```python
from build123d import *

# Parameters (mm, degrees)
SKETCH1_R           = 2.1
BOSS_EXTRUDE1_DEPTH = 65
SKETCH84_W          = 0.3
SKETCH84_H          = 5.4
BOSS_EXTRUDE6_DEPTH = 430
SKETCH85_W          = 26.589814492
SKETCH85_H          = 26.977421118
CUT_EXTRUDE59_DEPTH = 434.070721707
SKETCH86_W          = 10.5
SKETCH86_H          = 16.670499862
CUT_EXTRUDE60_DEPTH = 20
SKETCH88_W          = 63.871976351
SKETCH88_H          = 27.184970046
CUT_EXTRUDE62_DEPTH = 215
BOSS_EXTRUDE7_DEPTH = 195


with BuildPart() as part:
    # Sketch1 → Boss-Extrude1 (new body)
    with BuildSketch(Plane(origin=(0, 0, 0), x_dir=(0, 0, -1), z_dir=(1, 0, 0))):
        with BuildLine():
            Line((-10, 9), (-10, 3))
            Line((-10, 3), (-8, 3))
            Line((-8, 3), (-8, 6))
            Line((-8, 6), (-7.060660172, 6))
            Line((-7.060660172, 6), (-4, 2.939339828))
            Line((-4, 2.939339828), (-4, -2.939339828))
            Line((-4, -2.939339828), (-7.060660172, -6))
            Line((-7.060660172, -6), (-8, -6))
            Line((-8, -6), (-8, -3))
            Line((-8, -3), (-10, -3))
            Line((-10, -3), (-10, -9))
            ThreePointArc((-10, -9), (-9.707106781, -9.707106781), (-9, -10))
            Line((-9, -10), (-3, -10))
            Line((-3, -10), (-3, -8))
            Line((-3, -8), (-6, -8))
            Line((-6, -8), (-6, -7.060660172))
            Line((-6, -7.060660172), (-2.939339828, -4))
            Line((-2.939339828, -4), (2.939339828, -4))
            Line((2.939339828, -4), (6, -7.060660172))
            Line((6, -7.060660172), (6, -8))
            Line((6, -8), (3, -8))
            Line((3, -8), (3, -10))
            Line((3, -10), (9, -10))
            ThreePointArc((9, -10), (9.707106781, -9.707106781), (10, -9))
            Line((10, -9), (10, -3))
            Line((10, -3), (8, -3))
            Line((8, -3), (8, -6))
            Line((8, -6), (7.060660172, -6))
            Line((7.060660172, -6), (4, -2.939339828))
            Line((4, -2.939339828), (4, 2.939339828))
            Line((4, 2.939339828), (7.060660172, 6))
            Line((7.060660172, 6), (8, 6))
            Line((8, 6), (8, 3))
            Line((8, 3), (10, 3))
            Line((10, 3), (10, 9))
            ThreePointArc((10, 9), (9.707106781, 9.707106781), (9, 10))
            Line((9, 10), (3, 10))
            Line((3, 10), (3, 8))
            Line((3, 8), (6, 8))
            Line((6, 8), (6, 7.060660172))
            Line((6, 7.060660172), (2.939339828, 4))
            Line((2.939339828, 4), (-2.939339828, 4))
            Line((-2.939339828, 4), (-6, 7.060660172))
            Line((-6, 7.060660172), (-6, 8))
            Line((-6, 8), (-3, 8))
            Line((-3, 8), (-3, 10))
            Line((-3, 10), (-9, 10))
            ThreePointArc((-9, 10), (-9.707106781, 9.707106781), (-10, 9))
        make_face()
        Circle(SKETCH1_R, mode=Mode.SUBTRACT)
    extrude(amount=BOSS_EXTRUDE1_DEPTH)

    # Sketch85 → Cut-Extrude59 (cut, through all)
    with BuildSketch(Plane(origin=(65, 0, 0), x_dir=(0, 0, -1), z_dir=(1, 0, 0))):
        with Locations((1.176321583, -0.814927094)):
            Rectangle(SKETCH85_W, SKETCH85_H)
    extrude(amount=-CUT_EXTRUDE59_DEPTH, mode=Mode.SUBTRACT)


with BuildPart() as body_2:
    # Sketch84 → Boss-Extrude6 (new body)
    with BuildSketch(Plane(origin=(65, 0, 0), x_dir=(0, 0, -1), z_dir=(1, 0, 0))):
        Polygon((-10, -2.7), (-10, 2.7), (-10.5, 2.7), (-10.5, 5), (-20.5, 5), (-20.5, 0), (-40.5, 0), (-40.5, 5), (-50.5, 5), (-50.5, -5), (-10.5, -5), (-10.5, -2.7), align=None)
        Polygon((-7.18492424, 5.7), (-4.3, 2.81507576), (-4.3, -2.81507576), (-7.18492424, -5.7), (-7.7, -5.7), (-7.7, -2.7), (-9.7, -2.7), (-9.7, 2.7), (-7.7, 2.7), (-7.7, 5.7), align=None)
        with Locations((-9.85, 0)):
            Rectangle(SKETCH84_W, SKETCH84_H)
    extrude(amount=BOSS_EXTRUDE6_DEPTH)

    # Sketch86 → Cut-Extrude60 (cut)
    with BuildSketch(Plane.ZY.offset(-65)):
        with Locations((5.25, -0.117074477)):
            Rectangle(SKETCH86_W, SKETCH86_H)
    extrude(amount=-CUT_EXTRUDE60_DEPTH, mode=Mode.SUBTRACT)

    # Sketch88 → Cut-Extrude62 (cut)
    with BuildSketch(Plane(origin=(495, 0, 0), x_dir=(0, 0, -1), z_dir=(1, 0, 0))):
        with Locations((-29.280082041, 0.441796331)):
            Rectangle(SKETCH88_W, SKETCH88_H)
    extrude(amount=-CUT_EXTRUDE62_DEPTH, mode=Mode.SUBTRACT)

    # Sketch89 → Boss-Extrude7 (add)
    with BuildSketch(Plane(origin=(280, 0, 0), x_dir=(0, 0, -1), z_dir=(1, 0, 0))):
        Polygon((-10.7, 2.9), (-10.7, -2.9), (-7.9, -2.9), (-7.9, -5.9), (-7.102081528, -5.9), (-4.1, -2.897918472), (-4.1, 2.897918472), (-7.102081528, 5.9), (-7.9, 5.9), (-7.9, 2.9), align=None)
        Polygon((-10.5, 2.7), (-10.5, -2.7), (-7.7, -2.7), (-7.7, -5.7), (-7.18492424, -5.7), (-4.3, -2.81507576), (-4.3, 2.81507576), (-7.18492424, 5.7), (-7.7, 5.7), (-7.7, 2.7), align=None, mode=Mode.SUBTRACT)
    extrude(amount=-BOSS_EXTRUDE7_DEPTH)


solid = body_2.part
```
Build history of the part. All positions in model axes, mm. A direction names the side the tool comes from. Give positions to 0.01 mm unless a question says otherwise; leave off trailing zeros. Order: outer loops, then holes, each group sorted by start corner. A loop starts at its lowest first (then second) coordinate and runs counter-clockwise, first axis right, second up. Notation, with made-up numbers: M 61.25,32 L 120.25,32 A27 cw 120.25,49 Z; hole C 20,88.25 d5. An arc over 180 degrees is marked long. Write item = value, one per line. Start each with the question number.
(1) Slice it at C-C on z = 15. Write the cut outline in (x, y).
(2) Slice it at A-A on x = 133. Write the cut outline in (y, z).
(3) Slice it at B-B on z = 32.5. Write the cut outline in (x, y).
(4) Which spindle directions (+Z, -Z, +X, -X, +Y, -Y) get a long thin tool onto all of the face, cutting with end or side? Do faces 4 (the flat face through (171, 3, 20.5)), 5 (the flat face through (85, 0, 7)), 6 (the flat face through (171, 5, 15)). Say none if no direction does.
(5) Probe L1, parallel to Z at x = 166, y = 4; L2, parallel to Z at x = 240, y = 3; L3, parallel to Y at x = 106.5, z = 19. List the from-to ranges inside material, lowest first. Write a range as [from, to].
(6) Pin check, flat tips, straight feed: pin 1 Ø3 at (x, z) = (226, 46.5) entering from +Y; pin 2 Ø2 at (y, z) = (0.5, 36) entering from +X; pin 3 Ø1.5 at (x, z) = (94.5, 25) entering from -Y. Stop position of each tip, or through.
(7) Two-plate mould, pull along Z, no slides. Class faces 1 (the flat face through (65, -1, 31)), 2 (the flat face through (171, 2, 40.5)), 3 (the flat face through (184, 0, 4.1)): released by +Z, released by -Z, zero draft, split by the parting line, or undercut.
Responses:
q1.outline = M 65,-5 L 280,-5 L 280,5 L 65,5 Z
q2.outline = M -5.9,7.1 L -2.9,4.1 L 2.9,4.1 L 5.9,7.1 L 5.9,7.9 L 2.9,7.9 L 2.9,10.5 L 5,10.5 L 5,20.5 L 0,20.5 L 0,40.5 L 5,40.5 L 5,50.5 L -5,50.5 L -5,10.5 L -2.9,10.5 L -2.9,7.9 L -5.9,7.9 Z
q3.outline = M 65,-5 L 280,-5 L 280,0 L 65,0 Z
q4.face_4 = +X, -X, +Y
q4.face_5 = -Z, -X, +Y, -Y
q4.face_6 = +Z, +X, -X, +Y
q5.L1 = [5.2, 7.9], [10.5, 20.5], [40.5, 50.5]
q5.L2 = [4.2, 7.9], [10.5, 20.5], [40.5, 50.5]
q5.L3 = [-5, 5]
q6.pin_1 = 5
q6.pin_2 = 280
q6.pin_3 = -5
q7.face_1 = zero draft
q7.face_2 = undercut
q7.face_3 = released by -Z
